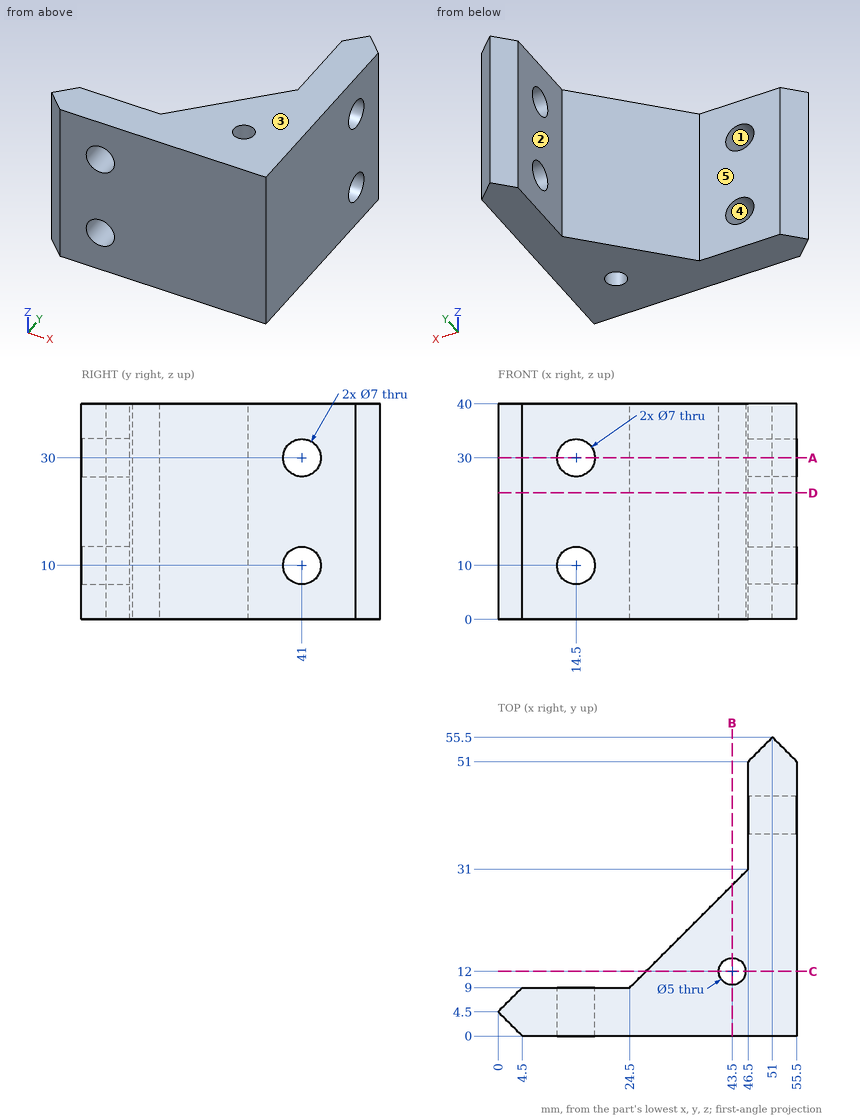
Input: dimensioned drawing with shaded views. Units: mm. Origin: part minimum x, y, z. A direction names the side the tool comes from. Coordinates: 2 decimals unless noted, no trailing zeros. Write each loop counter-clockwise with the first axis right and the second up, starting at its lowest first coordinate (ties: lowest second). Pieces come first, ordered by that corner, then holes. Notation, with made-up numbers: (22, -14.5) -> (73, -14.5) arc R22 cw to (73, 11.5) -> close; hole circle Ø7 at (-16.5, 23.25). An arc over 180 degrees is marked (long way). Return JSON: item names as keys, results as strings. Group by question number.
1) Section query C-C, the plane y = 12. Return loops of the section in (x, z), plus the area to 3 significant figures.
2) Ray query, line 1 along X through (y, z) = (11, 33.5); line 2 along Y through (x, z) = (22, 28); line 3 along X through (y, z) = (5.75, 30). Return the intervals inside material, ascending.
3) Set-up query: the marked faces 1 and 2. Return all of +Z, -Z, +X, -X, +Y, -Y with unobstructed straight access to the full face (end or side cutting, diameter ignored); none if empty.
4) Section query D-D, the plane z = 23.5. Return loops of the section in (x, y), plus the area to 3 significant figures.
5) Contact query for flat-ended pins moving along their axis: P1, Ø1.5, axis at x = 30.5, z = 11.5, coming from the +Y side; P2, Ø3, axis at x = 13.5, z = 9, coming from the +Y side; P3, Ø9, axis at y = 41, z = 30, coming from the -X side; P4, Ø4, axis at x = 21.5, z = 32, coming from the +Y side. Output: stop coordinate, or through.
6) Mould query, pull axis Z, two halves, no side actions, for the marked faces 3, 4 and 5. Classes: +Z half, -Z half, draft (parallel to the pull), parting line (faces both ways), or undercut.
7) Section query A-A, the plane z = 30. Return loops of the section in (x, y).
8) Section query B-B, the plane x = 43.5. Return loops of the section in (y, z), plus the area to 3 significant figures.
From the geometry:
{
 "1": {"outline": "(27.5, 0) -> (41, 0) -> (41, 40) -> (27.5, 40) -> close; (46, 0) -> (55.5, 0) -> (55.5, 40) -> (46, 40) -> close", "area": "920 mm²"},
 "2": {"line 1": "26.5 to 41.21, 45.79 to 55.5", "line 2": "0 to 9", "line 3": "1.25 to 11, 18 to 55.5"},
 "3": {"face 1": "+Y, -Y", "face 2": "+Z, -Z, -X, +Y"},
 "4": {"outline": "(0, 4.5) -> (4.5, 0) -> (55.5, 0) -> (55.5, 51) -> (51, 55.5) -> (46.5, 51) -> (46.5, 31) -> (24.5, 9) -> (4.5, 9) -> close; hole circle Ø5 at (43.5, 12)", "area": "1,100 mm²"},
 "5": {"P1": "y = 15.75", "P2": "through", "P3": "x = 46.5", "P4": "y = 9"},
 "6": {"face 3": "+Z half", "face 4": "undercut", "face 5": "draft"},
 "7": {"outline": "(0, 4.5) -> (4.5, 0) -> (11, 0) -> (11, 9) -> (4.5, 9) -> close; (18, 0) -> (55.5, 0) -> (55.5, 37.5) -> (46.5, 37.5) -> (46.5, 31) -> (24.5, 9) -> (18, 9) -> close; (46.5, 44.5) -> (55.5, 44.5) -> (55.5, 51) -> (51, 55.5) -> (46.5, 51) -> close; hole circle Ø5 at (43.5, 12)"},
 "8": {"outline": "(0, 0) -> (9.5, 0) -> (9.5, 40) -> (0, 40) -> close; (14.5, 0) -> (28, 0) -> (28, 40) -> (14.5, 40) -> close", "area": "920 mm²"}
}
